```python
from build123d import *

# Parameters (mm, degrees)
SKETCH1_W                      = 88.9
SKETCH1_H                      = 88.9
SKETCH1_W_2                    = 54.9
SKETCH1_H_2                    = 54.9
BOSS_EXTRUDE1_DEPTH            = 6.35
CHAMFER1_SIZE                  = 6.35
CBORE_FOR_M5_SHCS3_D           = 5.5
CBORE_FOR_M5_SHCS3_CBORE_D     = 10
CBORE_FOR_M5_SHCS3_CBORE_DEPTH = 5


with BuildPart() as part:
    # Sketch1 → Boss-Extrude1 (new body)
    with BuildSketch(Plane(origin=(0, 0, 0), x_dir=(1, 0, 0), z_dir=(0, 1, 0))):
        Rectangle(SKETCH1_W, SKETCH1_H)
        Rectangle(SKETCH1_W_2, SKETCH1_H_2, mode=Mode.SUBTRACT)
    extrude(amount=BOSS_EXTRUDE1_DEPTH)

    # Chamfer1
    chamfer1_edges = [part.edges().sort_by_distance(p)[0] for p in [
        (0, 6.35, 27.45),
        (27.45, 6.35, 0),
        (-27.45, 6.35, 0),
        (0, 6.35, -27.45),
    ]]
    chamfer(chamfer1_edges, length=CHAMFER1_SIZE - 0.0001)  # a hair under: the kernel refuses the full size

    # CBORE for M5 SHCS3 (through all)
    with Locations(Plane(origin=(0, 6.35, 0), x_dir=(1, 0, 0), z_dir=(0, 1, 0))):
        with Locations((-22.523488527, 38.45), (0, 38.45), (22.523488527, 38.45), (38.45, 22.523488527), (38.45, 0), (38.45, -22.523488527), (22.523488527, -38.45), (0, -38.45), (-22.523488527, -38.45), (-38.45, -22.523488527), (-38.45, 0), (-38.45, 22.523488527)):
            CounterBoreHole(CBORE_FOR_M5_SHCS3_D / 2, CBORE_FOR_M5_SHCS3_CBORE_D / 2, CBORE_FOR_M5_SHCS3_CBORE_DEPTH)


solid = part.part
```
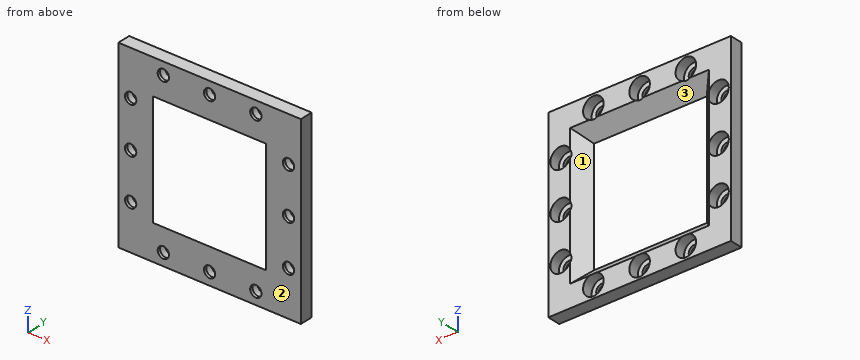
Input: part model. Units: mm. Frame: model coordinates. Face numbers are marked on the shaded views. Give positions to 0.01 mm unless a question says otherwise; leave off trailing zeros. Order: outer loops, then holes, each group sorted by start corner. A loop starts at its lowest first (then second) coordinate and runs counter-clockwise, first axis right, second up.
1. Mould query, pull axis Z, two halves, no side actions, for the marked faces 1, 2 and 3. Classes: released by +Z, released by -Z, zero draft, split by the parting line, or undercut.
Derived:
face 1: undercut
face 2: zero draft
face 3: undercut
2. Section C-C on y = 4.5. Give the number of separate pieces and of enclosed holes in the cut face, and give its area (3 significant figures).
Derived:
separate pieces: 1
enclosed holes: 13
area: 2,880 mm2
3. Section B-B on z = -38.45. Return the cut outline in (x, y).
Derived:
outline: (-44.45, 0) - (-25.27, 0) - (-25.27, 1.35) - (-27.52, 1.35) - (-27.52, 6.35) - (-44.45, 6.35) - close; (-19.77, 0) - (-2.75, 0) - (-2.75, 1.35) - (-5, 1.35) - (-5, 6.35) - (-17.52, 6.35) - (-17.52, 1.35) - (-19.77, 1.35) - close; (2.75, 0) - (19.77, 0) - (19.77, 1.35) - (17.52, 1.35) - (17.52, 6.35) - (5, 6.35) - (5, 1.35) - (2.75, 1.35) - close; (25.27, 0) - (44.45, 0) - (44.45, 6.35) - (27.52, 6.35) - (27.52, 1.35) - (25.27, 1.35) - close
4. Pin query (flat end, axial travel): pin 1 (5 mm diameter, centred on x = 23.5, z = -37.5, fed in from +Y). Return the tip coordinate at first contact, or that it passes through.
Derived:
pin 1: stops at y = 1.35
5. Material intervals for L1, parallel to Z at x = -38.45, y = 0.85; L2, parallel to Z at x = 38.45, y = 5.3, sorted ascending.
Derived:
L1: z = -44.45 to -25.27, -19.77 to -2.75, 2.75 to 19.77, 25.27 to 44.45
L2: z = -44.45 to -27.52, -17.52 to -5, 5 to 17.52, 27.52 to 44.45
6. Section A-A on x = -38.45. Return the cut outline in (y, z), and give its area (3 significant figures).
Derived:
outline: (0, -44.45) - (6.35, -44.45) - (6.35, -27.52) - (1.35, -27.52) - (1.35, -25.27) - (0, -25.27) - close; (0, -19.77) - (1.35, -19.77) - (1.35, -17.52) - (6.35, -17.52) - (6.35, -5) - (1.35, -5) - (1.35, -2.75) - (0, -2.75) - close; (0, 2.75) - (1.35, 2.75) - (1.35, 5) - (6.35, 5) - (6.35, 17.52) - (1.35, 17.52) - (1.35, 19.77) - (0, 19.77) - close; (0, 25.27) - (1.35, 25.27) - (1.35, 27.52) - (6.35, 27.52) - (6.35, 44.45) - (0, 44.45) - close
area: 392 mm2
